from build123d import *

# Parameters (mm, degrees)
SKETCH1_W                        = 32.131
SKETCH1_H                        = 25.4
BOSS_EXTRUDE1_DEPTH              = 32.131
SKETCH2_W                        = 1.27
SKETCH2_H                        = 32.131
SKETCH2_W_2                      = 32.131
SKETCH2_H_2                      = 1.27
CUT_EXTRUDE1_DEPTH               = 12.7
SKETCH3_R                        = 6.985
CUT_EXTRUDE2_DEPTH               = 1.27
F_10_0_1935_DIAMETER_HOLE6_D     = 4.9149
F_10_0_1935_DIAMETER_HOLE6_DEPTH = 7.62
F_10_0_1935_DIAMETER_HOLE6_TIP   = 1.476584928
F_10_0_1935_DIAMETER_HOLE7_D     = 4.9149
F_10_0_1935_DIAMETER_HOLE7_DEPTH = 7.62
F_10_0_1935_DIAMETER_HOLE7_TIP   = 1.476584928
F_10_0_1935_DIAMETER_HOLE8_D     = 4.9149
F_10_0_1935_DIAMETER_HOLE8_DEPTH = 7.62
F_10_0_1935_DIAMETER_HOLE8_TIP   = 1.476584928
F_10_0_1935_DIAMETER_HOLE9_D     = 4.9149
F_10_0_1935_DIAMETER_HOLE9_DEPTH = 7.62
F_10_0_1935_DIAMETER_HOLE9_TIP   = 1.476584928


with BuildPart() as part:
    # Sketch1 → Boss-Extrude1 (new body)
    with BuildSketch(Plane.XY):
        with Locations((0, 3.3655)):
            Rectangle(SKETCH1_W, SKETCH1_H)
    extrude(amount=BOSS_EXTRUDE1_DEPTH)

    # Sketch2 → Cut-Extrude1 (cut)
    with BuildSketch(Plane(origin=(0, 16.0655, 0), x_dir=(1, 0, 0), z_dir=(0, 1, 0))):
        with Locations((-4.7625, -16.0655)):
            Rectangle(SKETCH2_W, SKETCH2_H)
        with Locations((4.7625, -16.0655)):
            Rectangle(SKETCH2_W, SKETCH2_H)
        with Locations((0, -11.303)):
            Rectangle(SKETCH2_W_2, SKETCH2_H_2)
        with Locations((0, -20.828)):
            Rectangle(SKETCH2_W_2, SKETCH2_H_2)
    extrude(amount=-CUT_EXTRUDE1_DEPTH, mode=Mode.SUBTRACT)

    # Sketch3 → Cut-Extrude2 (cut)
    with BuildSketch(Plane(origin=(0, 16.0655, 0), x_dir=(1, 0, 0), z_dir=(0, 1, 0))):
        with Locations((0, -16.0655)):
            Circle(SKETCH3_R)
    extrude(amount=-CUT_EXTRUDE2_DEPTH, mode=Mode.SUBTRACT)

    # #10 (0.1935) Diameter Hole6
    with Locations(Plane.XY.offset(32.131)):
        with Locations((0, 0)):
            Hole(F_10_0_1935_DIAMETER_HOLE6_D / 2, depth=F_10_0_1935_DIAMETER_HOLE6_DEPTH)
            with Locations((0, 0, -(F_10_0_1935_DIAMETER_HOLE6_DEPTH + F_10_0_1935_DIAMETER_HOLE6_TIP / 2))):  # 118° drill point
                Cone(0, F_10_0_1935_DIAMETER_HOLE6_D / 2, F_10_0_1935_DIAMETER_HOLE6_TIP, mode=Mode.SUBTRACT)

    # #10 (0.1935) Diameter Hole7
    with Locations(Plane(origin=(0, 0, 0), x_dir=(-1, 0, 0), z_dir=(0, 0, -1))):
        with Locations((0, 0)):
            Hole(F_10_0_1935_DIAMETER_HOLE7_D / 2, depth=F_10_0_1935_DIAMETER_HOLE7_DEPTH)
            with Locations((0, 0, -(F_10_0_1935_DIAMETER_HOLE7_DEPTH + F_10_0_1935_DIAMETER_HOLE7_TIP / 2))):  # 118° drill point
                Cone(0, F_10_0_1935_DIAMETER_HOLE7_D / 2, F_10_0_1935_DIAMETER_HOLE7_TIP, mode=Mode.SUBTRACT)

    # #10 (0.1935) Diameter Hole8
    with Locations(Plane(origin=(16.0655, 0, 0), x_dir=(0, 0, -1), z_dir=(1, 0, 0))):
        with Locations((-16.0655, 0)):
            Hole(F_10_0_1935_DIAMETER_HOLE8_D / 2, depth=F_10_0_1935_DIAMETER_HOLE8_DEPTH)
            with Locations((0, 0, -(F_10_0_1935_DIAMETER_HOLE8_DEPTH + F_10_0_1935_DIAMETER_HOLE8_TIP / 2))):  # 118° drill point
                Cone(0, F_10_0_1935_DIAMETER_HOLE8_D / 2, F_10_0_1935_DIAMETER_HOLE8_TIP, mode=Mode.SUBTRACT)

    # #10 (0.1935) Diameter Hole9
    with Locations(Plane.ZY.offset(16.0655)):
        with Locations((16.0655, 0)):
            Hole(F_10_0_1935_DIAMETER_HOLE9_D / 2, depth=F_10_0_1935_DIAMETER_HOLE9_DEPTH)
            with Locations((0, 0, -(F_10_0_1935_DIAMETER_HOLE9_DEPTH + F_10_0_1935_DIAMETER_HOLE9_TIP / 2))):  # 118° drill point
                Cone(0, F_10_0_1935_DIAMETER_HOLE9_D / 2, F_10_0_1935_DIAMETER_HOLE9_TIP, mode=Mode.SUBTRACT)


solid = part.part
The listing builds one solid part. Answer for the finished solid, in the listing's coordinates (mm). A direction names the side the tool comes from. Round coordinates to 2 decimals unless told otherwise and drop trailing zeros. Order: outer loops, then holes, each group sorted by start corner. A loop starts at its lowest first (then second) coordinate and runs counter-clockwise, first axis right, second up. Notation, with made-up numbers: M 85.25,-32 L 136.25,-32 A27 cw 136.25,-8 Z; hole C 26,-34.75 d3. An arc over 180 degrees is marked long. Answer in a Markdown table with one row per item. Add a question column.
1) The part is cut by section A-A on z = 27.5. Determine the outline of the cut face in (x, y).
2) Which of the six approach directions +Z, -Z, +X, -X, +Y, -Y give full straight-line access (tool end or side, diameter ignored) to faces 4 (the face through (0, 16.066, 5)), 5 (the face through (0, 14.796, 16)), 6 (the face through (5.398, 10, 5)), 7 (the face through (-11, 10, 20.193)), 8 (the face through (1.13, -2.18, 3.86))?
3) Consider line 1 along Z through (x, y) = (7.5, 3.5); line 2 along X through (y, z) = (14, 15); line 3 along X through (y, z) = (0, 2.25). Determine where each line is inside the solid, lowest interval first. Write a range as from..to.
4) Determine the mould class of faces 1 (the face through (11, 10, 11.938)), 2 (the face through (6, 14.796, 16)), 3 (the face through (11, 16.066, 5)) for opening direction Z: pulls with the +Z half, pulls with the -Z half, needs draft (parallel to the pull), parting line crosses it, or undercut.
5) A flat-ended cylindrical pin translates along its axis: pin 1 Ø0.5 at (x, z) = (6, 16.5) entering from +Y. Find the tip coordinate at first contact, or state that the pin passes through.
6) The part is cut by section B-B on x = -11. Determine the outline of the cut face in (y, z), plus the area to 3 significant figures.
Findings below:
| question | item | result |
|---|---|---|
| 1 | outline | M -16.07,-9.33 L 16.07,-9.33 L 16.07,16.07 L 5.4,16.07 L 5.4,3.37 L 4.13,3.37 L 4.13,16.07 L -4.13,16.07 L -4.13,3.37 L -5.4,3.37 L -5.4,16.07 L -16.07,16.07 Z; hole C 0,0 d4.91 |
| 2 | face 4 | +Z, -Z, +X, -X, +Y |
| 2 | face 5 | +Y |
| 2 | face 6 | +Z, -Z, +Y |
| 2 | face 7 | +X, -X, +Y |
| 2 | face 8 | -Z |
| 3 | line 1 | z = 0..10.67, 11.94..20.19, 21.46..32.13 |
| 3 | line 2 | x = -16.07..-5.4, -4.13..4.13, 5.4..16.07 |
| 3 | line 3 | x = -16.07..-2.46, 2.46..16.07 |
| 4 | face 1 | undercut |
| 4 | face 2 | undercut |
| 4 | face 3 | needs draft |
| 5 | pin 1 | stops at y = 14.8 |
| 6 | outline | M -9.33,0 L 16.07,0 L 16.07,10.67 L 3.37,10.67 L 3.37,11.94 L 16.07,11.94 L 16.07,20.19 L 3.37,20.19 L 3.37,21.46 L 16.07,21.46 L 16.07,32.13 L -9.33,32.13 Z; hole C 0,16.07 d4.91 |
| 6 | area | 765 mm² |
